Geometry check sheet. Reference: the model listing, model coordinates, mm. A direction names the side the tool comes from. Give positions to 0.01 mm unless a question says otherwise; leave off trailing zeros. Loops run counter-clockwise (first coordinate to the right, second up) from the corner with the lowest first, then second, coordinate; pieces in that order, holes last. Notation, with made-up numbers: (70, 9) -> (91, 9) arc R20 ccw to (91, 46) -> close; hole circle Ø3 at (-7.5, 85). An arc over 180 degrees is marked (long way). Write item = value, one per line.
```python
from build123d import *

# Parameters (mm, degrees)
BASE_DEPTH         = 3.81
METRIC_HOLES_REACH = 20.88
SKETCH3_R          = 2.032
SKETCH3_R_2        = 1.905
SKETCH4_R          = 3.4925
CUT_EXTRUDE2_DEPTH = 2.54


with BuildPart() as part:
    # Sketch2 → base (new body)
    with BuildSketch(Plane(origin=(0, 0, 0), x_dir=(0, 1, 0), z_dir=(0, 0, 1))):
        with BuildLine():
            Line((0, 5.08), (12.7, 5.08))
            ThreePointArc((12.7, 5.08), (17.78, 0), (12.7, -5.08))
            Line((12.7, -5.08), (0, -5.08))
            ThreePointArc((0, -5.08), (-5.08, 0), (0, 5.08))
        make_face()
    extrude(amount=BASE_DEPTH)

    # Sketch3 → metric_holes (cut, up to next)
    with BuildSketch(Plane.XY.offset(3.81), mode=Mode.PRIVATE) as metric_holes_sk1:
        Circle(SKETCH3_R)
    metric_holes_tool1 = extrude(metric_holes_sk1.sketch, amount=-METRIC_HOLES_REACH, mode=Mode.PRIVATE) & part.part
    # Sketch3 → metric_holes (cut, up to next)
    with BuildSketch(Plane.XY.offset(3.81), mode=Mode.PRIVATE) as metric_holes_sk2:
        with Locations((0, 12.7)):
            Circle(SKETCH3_R_2)
    metric_holes_tool2 = extrude(metric_holes_sk2.sketch, amount=-METRIC_HOLES_REACH, mode=Mode.PRIVATE) & part.part
    add(metric_holes_tool1.solids().sort_by_distance((0, 0, 3.81))[0], mode=Mode.SUBTRACT)
    add(metric_holes_tool2.solids().sort_by_distance((0, 12.7, 3.81))[0], mode=Mode.SUBTRACT)

    # Sketch4 → Cut-Extrude2 (cut)
    with BuildSketch(Plane.XY.offset(3.81)):
        Circle(SKETCH4_R)
    extrude(amount=-CUT_EXTRUDE2_DEPTH, mode=Mode.SUBTRACT)


solid = part.part
```
Item 1: Section check D-D, the plane z = 1.75. Record the cut outline in (x, y) (1 decimal).
Answer:
outline = (-5.1, 0) arc R5.1 ccw to (5.1, 0) -> (5.1, 12.7) arc R5.1 ccw to (-5.1, 12.7) -> close; hole circle Ø7 at (0, 0); hole circle Ø3.8 at (0, 12.7)
Item 2: Draft check along X on faces 1 (the flat face through (0, 7, 3.81)), 2 (the cylindrical face through (-0.41, 10.84, 1.93)), 3 (the flat face through (5.08, 6, 2)). Enter one of: +X half, -X half, draft (parallel to the pull), parting line (faces both ways), or undercut.
Answer:
face_1 = draft
face_2 = undercut
face_3 = +X half
Item 3: Section check B-B, the plane y = 11.25. Record the cut outline in (x, z).
Answer:
outline = (-5.08, 0) -> (-1.24, 0) -> (-1.24, 3.81) -> (-5.08, 3.81) -> close; (1.24, 0) -> (5.08, 0) -> (5.08, 3.81) -> (1.24, 3.81) -> close
Item 4: Gauge pin test, flat ends, axial feed: pin 1 (2 mm diameter, centred on x = 1, y = -0.5, fed in from +Z); pin 2 (1.5 mm diameter, centred on x = 3.5, z = 2.5, fed in from +Y); pin 3 (3.5 mm diameter, centred on x = 0, y = 0, fed in from -Z). Record the tip position at first contact, or that the pin passes through.
Answer:
pin_1 = 1.27
pin_2 = 16.97
pin_3 = through
Item 5: Section check A-A, the plane x = 0. Record the cut outline in (y, z) (1 decimal), plus the area to 3 significant figures.
Answer:
outline = (-5.1, 0) -> (-2, 0) -> (-2, 1.3) -> (-3.5, 1.3) -> (-3.5, 3.8) -> (-5.1, 3.8) -> close; (2, 0) -> (10.8, 0) -> (10.8, 3.8) -> (3.5, 3.8) -> (3.5, 1.3) -> (2, 1.3) -> close; (14.6, 0) -> (17.8, 0) -> (17.8, 3.8) -> (14.6, 3.8) -> close
area = 49.7 mm^2
Item 6: Section check C-C, the plane z = 0.8. Record the cut outline in (x, y) (3 decimals), plus the area to 3 significant figures.
Answer:
outline = (-5.08, 0) arc R5.08 ccw to (5.08, 0) -> (5.08, 12.7) arc R5.08 ccw to (-5.08, 12.7) -> close; hole circle Ø4.064 at (0, 0); hole circle Ø3.81 at (0, 12.7)
area = 186 mm^2
Item 7: Thickness scan on L1, parallel to Y at x = 0, z = 2.25 (1 decimal); L2, parallel to Y at x = 0, z = 0.35 (3 decimals); L3, parallel to Z at x = 1.75, y = 1.5. Record the ranges inside material, lowest first. Write a range as [from, to].
Answer:
L1 = [-5.1, -3.5], [3.5, 10.8], [14.6, 17.8]
L2 = [-5.08, -2.032], [2.032, 10.795], [14.605, 17.78]
L3 = [0, 1.27]
Item 8: Tool access check on faces 4 (the cylindrical face through (-0.455, 3.463, 2.558)), 5 (the flat face through (0, 7, 0)). Record the directions out of +Z, -Z, +X, -X, +Y, -Y that give a thin tool (end or side, any length) a straight path to the whole face; none if there is none.
Answer:
face_4 = +Z
face_5 = -Z, +X, -X, +Y, -Y
